Geometry check sheet. Reference: the model listing, model coordinates, mm. A direction names the side the tool comes from. Round coordinates to 2 decimals unless told otherwise and drop trailing zeros. Write each loop counter-clockwise with the first axis right and the second up, starting at its lowest first coordinate (ties: lowest second). Pieces come first, ordered by that corner, then holes. Notation, with made-up numbers: M 83,31.25 L 130,31.25 A23 ccw 130,51.25 Z; hole C 62.25,-12.5 d3. An arc over 180 degrees is marked long. Use a Markdown table: item, result.
```python
from build123d import *

# Parameters (mm, degrees)
F0_R     = 47.56572
F1_DEPTH = 104.648
F2_R     = 27.682739
F3_DEPTH = 25.4
F4_W     = 48.33358
F4_H     = 33.992838
F5_DEPTH = 254


with BuildPart() as f1:
    # F0 (on Top) → F1 (new body)
    with BuildSketch(Plane.XY):
        Circle(F0_R)
    extrude(amount=F1_DEPTH)

    # F2 (on face) → F3 (join)
    with BuildSketch(Plane.XY.offset(104.648)):
        with Locations((-4.464226, 0)):
            Circle(F2_R)
    extrude(amount=F3_DEPTH)

    # F4 (on face) → F5 (join)
    with BuildSketch(Plane.XY.offset(130.048)):
        with Locations((-7.980175, -16.996419)):
            Rectangle(F4_W, F4_H)
    extrude(amount=F5_DEPTH)


solid = f1.part
```
Item 1: Cross-section at D-D, the plane y = -8. Record the cut outline in (x, z), and give its area (3 significant figures).
Outcome:
| item | result |
|---|---|
| outline | M -46.89,0 L 46.89,0 L 46.89,104.65 L 22.04,104.65 L 22.04,130.05 L 16.19,130.05 L 16.19,384.05 L -32.15,384.05 L -32.15,130.05 L -30.97,130.05 L -30.97,104.65 L -46.89,104.65 Z |
| area | 23,400 mm2 |
Item 2: Cross-section at A-A, the plane x = 6. Record the cut outline in (y, z), and give its area (3 significant figures).
Outcome:
| item | result |
|---|---|
| outline | M -47.19,0 L 47.19,0 L 47.19,104.65 L 25.63,104.65 L 25.63,130.05 L 0,130.05 L 0,384.05 L -33.99,384.05 L -33.99,130.05 L -25.63,130.05 L -25.63,104.65 L -47.19,104.65 Z |
| area | 19,800 mm2 |
Item 3: Cross-section at C-C, the plane z = 263. Record the cut outline in (x, y).
Outcome:
| item | result |
|---|---|
| outline | M -32.15,-33.99 L 16.19,-33.99 L 16.19,0 L -32.15,0 Z |
Item 4: Cross-section at B-B, the plane y = 11. Record the cut outline in (x, z).
Outcome:
| item | result |
|---|---|
| outline | M -46.28,0 L 46.28,0 L 46.28,104.65 L 20.94,104.65 L 20.94,130.05 L -29.87,130.05 L -29.87,104.65 L -46.28,104.65 Z |
Item 5: Access from +Z, -Z, +X, -X, +Y, -Y to the whole of each face (thin tool, end or side, straight path). Record for faces 1 (the face through (16.187, -17, 255)), 2 (the face through (10.42, 23.34, 117.17)), 3 (the face through (-32.147, -17, 255)), 4 (the face through (-8, -33.993, 255)).
Outcome:
| item | result |
|---|---|
| face 1 | +Z, +X, +Y, -Y |
| face 2 | none |
| face 3 | +Z, -X, +Y, -Y |
| face 4 | +Z, +X, -X, -Y |
Item 6: Material ranges on line 1 along X through (y, z) = (1, 86); line 2 along Z through (x, y) = (-30.5, 21); line 3 along Z through (x, y) = (-1, 1), recorded low to high. Write a range as from..to.
Outcome:
| item | result |
|---|---|
| line 1 | x = -47.56..47.56 |
| line 2 | z = 0..104.65 |
| line 3 | z = 0..130.05 |
Item 7: Go/stop test with flat-tipped pins: pin 1 (10 mm diameter, centred on y = -14.5, z = 304.5, fed in from +X); pin 2 (6 mm diameter, centred on x = -17, z = 302, fed in from -Y); pin 3 (1.5 mm diameter, centred on x = -36.5, y = 25, fed in from +Z). Record where each tip stops, or that it passes through.
Outcome:
| item | result |
|---|---|
| pin 1 | stops at x = 16.19 |
| pin 2 | stops at y = -33.99 |
| pin 3 | stops at z = 104.65 |
Item 8: Mould release check, pull along Z, two halves, no side actions. Record for faces 5 (the face through (-8, 0, 255)), 6 (the face through (-1, 1, 0)), 7 (the face through (-12, -27, 130.048)): +Z half, -Z half, draft (parallel to the pull), parting line (faces both ways), or undercut.
Outcome:
| item | result |
|---|---|
| face 5 | draft |
| face 6 | -Z half |
| face 7 | undercut |
